Autodesk Inventor part; units mm, degrees
ref_plane "YZ Plane" through (0, 0, 0) normal (1, 0, 0) x (0, 1, 0)
ref_plane "XZ Plane" through (0, 0, 0) normal (0, 1, 0) x (-1, 0, 0)
ref_plane "XY Plane" through (0, 0, 0) normal (0, 0, 1) x (1, 0, 0)
sketch "スケッチ1" plane through (0, 0, 0) normal (0, 1, 0) x (-1, 0, 0)
  line L0 (1.7321, -3) -> (-1.7321, -3)
  line L1 (-1.7321, -3) -> (-3.4641, 0)
  line L2 (-3.4641, 0) -> (-1.7321, 3)
  line L3 (-1.7321, 3) -> (1.7321, 3)
  line L4 (1.7321, 3) -> (3.4641, 0)
  line L5 (3.4641, 0) -> (1.7321, -3)
  line L6 (1.7321, -3) -> (-1.7321, 3) construction
  line L7 (-3.4641, 0) -> (3.4641, 0) construction
  line L8 (-1.7321, -3) -> (1.7321, 3) construction
  point P0 (0, 0)
  point P1 (0, 0)
  point P2 (0, 0)
  dimension "d0" = 6
extrude "押し出し1" add sketch "スケッチ1" along normal blind 10
sketch "スケッチ2" plane through (0, 10, 0) normal (0, 1, 0) x (1, 0, 0)
  point P0 (0, 0)
  point P1 (0, 0)
hole "穴1" at (0, 10, 0) direction (0, -1, 0) diameter 2.459 depth 4.8
sketch "スケッチ3" plane through (0, 0, 0) normal (0, -1, 0) x (1, 0, 0)
  circle A0 centre (0, 0) radius 1.5
  dimension "d10" = 3
extrude "押し出し2" add sketch "スケッチ3" along normal blind 5
thread "ねじ1"
properties part number "Spacer10mm" material "アセタール樹脂、黒"
Verification items for the finished model (mm, model axes). A direction names the side the tool comes from. Round coordinates to 2 decimals unless told otherwise and drop trailing zeros. Write each loop counter-clockwise with the first axis right and the second up, starting at its lowest first coordinate (ties: lowest second). Pieces come first, ordered by that corner, then holes. Notation, with made-up numbers: (44.25, 36) - (65.25, 36) arc R13 cw to (65.25, 44) - close; hole circle Ø5 at (85.5, -6). An arc over 180 degrees is marked (long way). Answer as a JSON object with one key per item and string values. Group by question number.
Q1. Section check C-C, the plane z = -1. Enter the section's corners in (x, y).
Q2. Tool access check on faces 5 (the flat face through (-1.5, 0, 0.7)), 6 (the flat face through (-1.5, 10, 0)). Record the directions out of +Z, -Z, +X, -X, +Y, -Y that give a thin tool (end or side, any length) a straight path to the whole face; none if there is none.
Q3. Mould release check, pull along X, two halves, no side actions. Record for faces 1 (the flat face through (0, 5.2, 0)), 2 (the flat face through (0, 5, 3)), 3 (the cylindrical face through (-1.5, -2.46, -0.07)), 4 (the cylindrical face through (0.748, 7.566, -0.976)): released by +X, released by -X, zero draft, split by the parting line, or undercut.
Q4. Section check D-D, the plane y = 4.25. Enter the section's corners in (x, z).
Q5. Section check B-B, the plane x = 0. Enter the section's corners in (y, z), plus the area to 3 significant figures.
Q6. Go/stop test with flat-tipped pins: pin 1 Ø0.7 at (x, z) = (-0.5, 0) entering from +Y; pin 2 Ø2 at (y, z) = (2.5, 0.5) entering from +X. Record where each tip stops, or that it passes through.
Q7. Section check A-A, the plane y = 7.5. Enter the section's corners in (x, z).
Q8. Thickness scan on line 1 (Z direction, x = 0, y = 6.95); line 2 (Y direction, x = -0.25, z = -1.6); line 3 (Z direction, x = 0, y = -1). Record the ranges inside material, lowest first.
Found:
{
 "1": {"outline": "(-2.89, 0) - (-1.12, 0) - (-1.12, -5) - (1.12, -5) - (1.12, 0) - (2.89, 0) - (2.89, 10) - (0.72, 10) - (0.72, 5.2) - (-0.72, 5.2) - (-0.72, 10) - (-2.89, 10) - close"},
 "2": {"face 5": "-Y", "face 6": "+Z, -Z, +X, -X, +Y"},
 "3": {"face 1": "undercut", "face 2": "zero draft", "face 3": "split by the parting line", "face 4": "undercut"},
 "4": {"outline": "(-3.46, 0) - (-1.73, -3) - (1.73, -3) - (3.46, 0) - (1.73, 3) - (-1.73, 3) - close"},
 "5": {"outline": "(-5, -1.5) - (0, -1.5) - (0, -3) - (10, -3) - (10, -1.23) - (5.2, -1.23) - (5.2, 1.23) - (10, 1.23) - (10, 3) - (0, 3) - (0, 1.5) - (-5, 1.5) - close", "area": "63.2 mm^2"},
 "6": {"pin 1": "stops at y = 5.2", "pin 2": "stops at x = 3.46"},
 "7": {"outline": "(-3.46, 0) - (-1.73, -3) - (1.73, -3) - (3.46, 0) - (1.73, 3) - (-1.73, 3) - close; hole circle Ø2.46 at (0, 0)"},
 "8": {"line 1": "z = -3 to -1.23, 1.23 to 3", "line 2": "y = 0 to 10", "line 3": "z = -1.5 to 1.5"}
}
